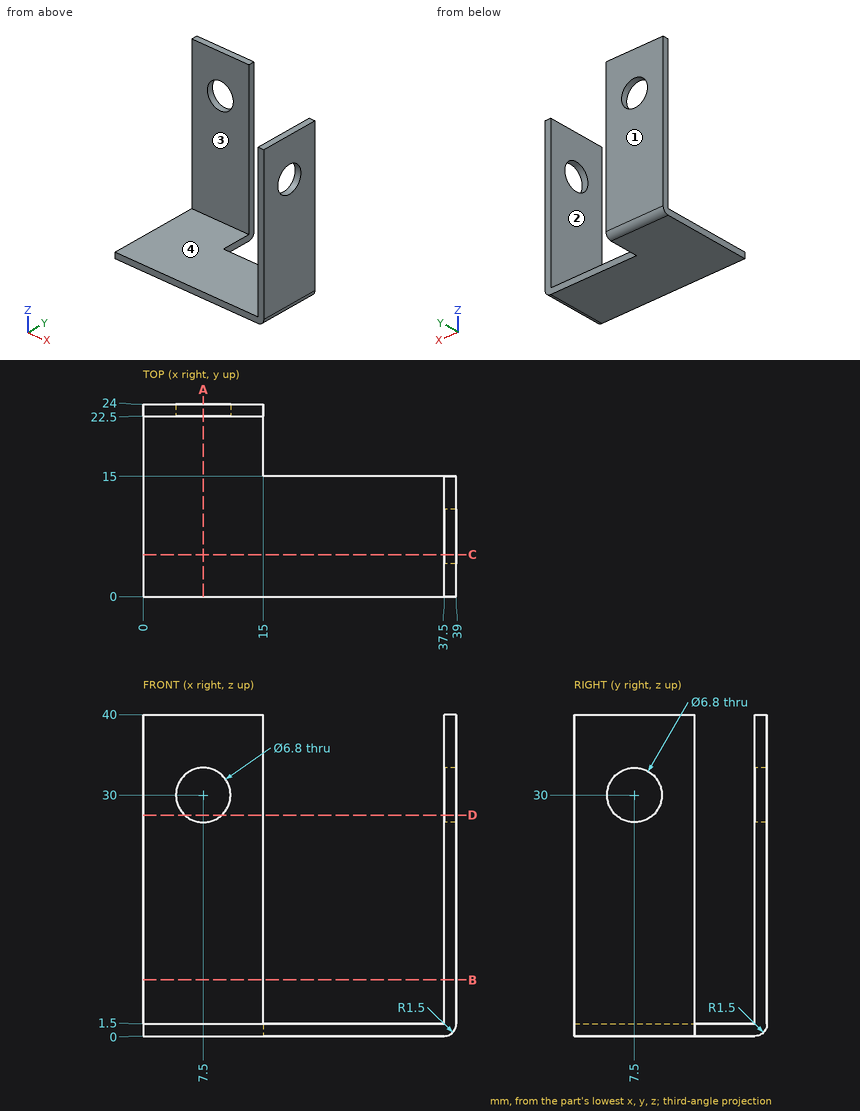
Could you check a few things on this drawing? It's one solid part, dimensions in mm from its lowest x, y, z. A direction names the side the tool comes from. Give positions to 0.01 mm unless a question says otherwise; leave off trailing zeros. Loops run counter-clockwise (first coordinate to the right, second up) from the corner with the lowest first, then second, coordinate; pieces in that order, holes last. Notation, with made-up numbers: M 46.25,57.5 L 84.25,57.5 A6 ccw 84.25,61.5 Z; hole C 74,55 d3. An arc over 180 degrees is marked long. Answer as a JSON object with one key per item and string values.
Q1. Suppose I cut it at D-D, the plane z = 27.5. List the corners of the cut face in (x, y) for me.
Values found:
{"outline": "M 0,22.5 L 5.2,22.5 L 5.2,24 L 0,24 Z; M 9.8,22.5 L 15,22.5 L 15,24 L 9.8,24 Z; M 37.5,0 L 39,0 L 39,5.2 L 37.5,5.2 Z; M 37.5,9.8 L 39,9.8 L 39,15 L 37.5,15 Z"}
Q2. For the marked faces 1, 2, 3 and 4, which set-ups out of +Z, -Z, +X, -X, +Y, -Y let a thin tool reach every point of the face, with its end or its side?
Values found:
{"face 1": "+Z, -Z, +X, -X, +Y", "face 2": "+Z, -X, +Y, -Y", "face 3": "+Z, +X, -X, -Y", "face 4": "+Z, -X, -Y"}
Q3. For P1, Ø4, axis at y = 7.5, z = 30, coming from the +X side; P2, Ø8, axis at x = 7.5, z = 30, coming from the +Y side; P3, Ø1, axis at y = 4.5, z = 9.5, coming from the -X side; P4, Ø2, axis at x = 15, y = 4.5, coming from the +Z side, each with a flat end and sliding along its axis, tell me the tip position at first contact or that it passes through.
Values found:
{"P1": "passes through", "P2": "stops at y = 24", "P3": "stops at x = 37.5", "P4": "stops at z = 1.5"}
Q4. Suppose I cut it at B-B, the plane z = 7. List the corners of the cut face in (x, y) for me.
Values found:
{"outline": "M 0,22.5 L 15,22.5 L 15,24 L 0,24 Z; M 37.5,0 L 39,0 L 39,15 L 37.5,15 Z"}
Q5. Suppose I cut it at C-C, the plane y = 5.25. List the corners of the cut face in (x, z) for me, plus the area to 3 significant figures.
Values found:
{"outline": "M 0,0 L 37.5,0 A1.5 ccw 39,1.5 L 39,27.45 L 37.5,27.45 L 37.5,1.5 L 0,1.5 Z; M 37.5,32.55 L 39,32.55 L 39,40 L 37.5,40 Z", "area": "108 mm²"}
Q6. If I drill on probe 1 along X at (y, z) = (23.1, 30); probe 2 along X at (y, z) = (5, 7.5), over which ranges is the centre line in solid material (lowest first)? Write a range as [from, to].
Values found:
{"probe 1": "x = [0, 4.1], [10.9, 15]", "probe 2": "x = [37.5, 39]"}
Q7. Suppose I cut it at A-A, the plane x = 7.5. List the corners of the cut face in (y, z) for me, plus the area to 3 significant figures.
Values found:
{"outline": "M 0,0 L 22.5,0 A1.5 ccw 24,1.5 L 24,26.6 L 22.5,26.6 L 22.5,1.5 L 0,1.5 Z; M 22.5,33.4 L 24,33.4 L 24,40 L 22.5,40 Z", "area": "83.1 mm²"}
